```python
from build123d import *

# Parameters (mm, degrees)
CROQUIS1_W              = 16
CROQUIS1_H              = 23.2
CROQUIS1_R              = 7
CROQUIS1_R_2            = 3
CROQUIS1_R_3            = 1.4
SALIENTE_EXTRUIR1_DEPTH = 30


with BuildPart() as part:
    # Croquis1 → Saliente-Extruir1 (new body)
    with BuildSketch(Plane.XZ.offset(21.216878831)):
        with Locations((-34.53076768, 9.025)):
            Rectangle(CROQUIS1_W, CROQUIS1_H)
        with Locations(Location((-34.53076768, 12.425, 0), (0, 0, 270))):
            Circle(CROQUIS1_R, mode=Mode.SUBTRACT)
        with Locations(Location((-38.83076768, 1.625, 0), (0, 0, 270))):
            Circle(CROQUIS1_R_2, mode=Mode.SUBTRACT)
        with Locations(Location((-28.53076768, 4.325, 0), (0, 0, 270))):
            Circle(CROQUIS1_R_3, mode=Mode.SUBTRACT)
    extrude(amount=-SALIENTE_EXTRUIR1_DEPTH)


solid = part.part
```
Can you work these out from the model? Positions are in its coordinate system, mm. Coordinates: 2 decimals unless noted, no trailing zeros. Loops run counter-clockwise (first coordinate to the right, second up) from the corner with the lowest first, then second, coordinate; pieces in that order, holes last.
Item 1: Please list where these lines run through material, in increasing order: L1, parallel to Z at x = -38, y = -4.75 (3 decimals); L2, parallel to Z at x = -40.5, y = -10.25 (3 decimals); L3, parallel to X at y = 1.75, z = 9.
Answers below:
L1: z = -2.575 to -1.258, 4.508 to 6.345, 18.505 to 20.625
L2: z = -2.575 to -0.868, 4.118 to 8.769, 16.081 to 20.625
L3: x = -42.53 to -40.64, -28.43 to -26.53
Item 2: Suppose I cut it at C-C (x = -38). Please give me the cut outline in (y, z) (3 decimals), then the cut area to 3 significant figures.
Answers below:
outline: (-21.217, -2.575) - (8.783, -2.575) - (8.783, -1.258) - (-21.217, -1.258) - close; (-21.217, 4.508) - (8.783, 4.508) - (8.783, 6.345) - (-21.217, 6.345) - close; (-21.217, 18.505) - (8.783, 18.505) - (8.783, 20.625) - (-21.217, 20.625) - close
area: 158 mm2
Item 3: Suppose I cut it at A-A (z = 15). Please give me the cut outline in (x, y).
Answers below:
outline: (-42.53, -21.22) - (-41.04, -21.22) - (-41.04, 8.78) - (-42.53, 8.78) - close; (-28.02, -21.22) - (-26.53, -21.22) - (-26.53, 8.78) - (-28.02, 8.78) - close
Item 4: Suppose I cut it at D-D (y = -11). Please give me the cut outline in (x, z) (3 decimals).
Answers below:
outline: (-42.531, -2.575) - (-26.531, -2.575) - (-26.531, 20.625) - (-42.531, 20.625) - close; hole circle Ø6 at (-38.831, 1.625); hole circle Ø14 at (-34.531, 12.425); hole circle Ø2.8 at (-28.531, 4.325)
Item 5: Suppose I cut it at B-B (x = -30.75). Please give me the cut outline in (y, z) (3 decimals).
Answers below:
outline: (-21.217, -2.575) - (8.783, -2.575) - (8.783, 6.534) - (-21.217, 6.534) - close; (-21.217, 18.316) - (8.783, 18.316) - (8.783, 20.625) - (-21.217, 20.625) - close
Item 6: If we mould it in two halves opening along X, with no side actions, what happens to faces 1 (the face through (-35, -21.217, 4)), 2 (the face through (-34.22, -6.43, 19.42)), 3 (the face through (-42.531, -6, 9))? For each: released by +X, released by -X, zero draft, split by the parting line, or undercut.
Answers below:
face 1: zero draft
face 2: undercut
face 3: released by -X
